from build123d import *

# Parameters (mm, degrees)
SKETCH4_W                         = 50
SKETCH4_H                         = 40
BOSS_EXTRUDE2_DEPTH               = 15
O_0_316_DIAMETER_HOLE1_AT_2_COUNT = 2
O_0_316_DIAMETER_HOLE1_AT_2_PITCH = 24
SKETCH10_W                        = 50
SKETCH10_H                        = 41.95
BOSS_EXTRUDE3_DEPTH               = 15
SKETCH12_W                        = 50
SKETCH12_H                        = 10
BOSS_EXTRUDE5_DEPTH               = 15
BOSS_EXTRUDE4_REACH               = 94.649
SKETCH11_W                        = 100
SKETCH11_H                        = 23.7
BOSS_EXTRUDE4_DIRECTION_2_DEPTH   = 25.4
O_0_316_DIAMETER_HOLE2_AT_2_COUNT = 2
O_0_316_DIAMETER_HOLE2_AT_2_PITCH = 25
O_0_316_DIAMETER_HOLE2_AT_3_COUNT = 2
O_0_316_DIAMETER_HOLE2_AT_3_PITCH = 50
O_0_316_DIAMETER_HOLE2_AT_4_COUNT = 2
O_0_316_DIAMETER_HOLE2_AT_4_PITCH = 75
CUT_EXTRUDE1_START                = -25.4
SKETCH13_R                        = 5.8
SKETCH13_R_2                      = 4.0132
CUT_EXTRUDE1_DEPTH                = 25.4
CHAMFER3_SIZE2                    = 25.4
CHAMFER3_SIZE                     = 14.664696837
FILLET1_R                         = 10


# Some blends are built 0.0001 mm under size
with BuildPart() as part:
    # Sketch4 → Boss-Extrude2 (new body)
    with BuildSketch(Plane(origin=(0, 0, 5), x_dir=(-1, 0, 0), z_dir=(0, 0, -1))):
        with Locations((6.635038983, -19.8)):
            Rectangle(SKETCH4_W, SKETCH4_H)
    extrude(amount=BOSS_EXTRUDE2_DEPTH)

    # Sketch9 → O (0.316) Diameter Hole1 (revolve, cut)
    with BuildSketch(Plane(origin=(-18.635038983, -19.8, 5), x_dir=(0, -1, 0), z_dir=(1, 0, 0))):
        Polygon((0, 0), (0, 15), (4.0132, 15), (4.0132, 6.350000732), (4.457235307, 0), align=None)
    o_0_316_diameter_hole1 = revolve(axis=Axis((-18.635038983, -19.8, 11.35), (0, 0, -1)), mode=Mode.SUBTRACT)

    # O (0.316) Diameter Hole1 at 2: O (0.316) Diameter Hole1 ×2
    with Locations(*[(i * O_0_316_DIAMETER_HOLE1_AT_2_PITCH, 0, 0) for i in range(1, O_0_316_DIAMETER_HOLE1_AT_2_COUNT)]):
        add(o_0_316_diameter_hole1, mode=Mode.SUBTRACT)

    # Sketch10 → Boss-Extrude3 (add)
    with BuildSketch(Plane(origin=(0, 0, -10), x_dir=(-1, 0, 0), z_dir=(0, 0, -1))):
        with Locations((6.635038983, -60.775)):
            Rectangle(SKETCH10_W, SKETCH10_H)
    extrude(amount=-BOSS_EXTRUDE3_DEPTH)

    # Sketch12 → Boss-Extrude5 (add)
    with BuildSketch(Plane.XY.offset(5)):
        with Locations((-6.635038983, -44.8)):
            Rectangle(SKETCH12_W, SKETCH12_H)
    extrude(amount=BOSS_EXTRUDE5_DEPTH)

    # Boss-Extrude4: up to this face of the body (flat: up to its plane)
    boss_extrude4_end = Plane(part.part.faces().sort_by_distance((-6.635038983, -19.8, 5))[0])
    # Sketch11 → Boss-Extrude4 (add, up to the picked face)
    with BuildSketch(Plane(origin=(0, 0, -10), x_dir=(-1, 0, 0), z_dir=(0, 0, -1)), mode=Mode.PRIVATE) as boss_extrude4_sk1:
        with Locations((-18.364961017, -69.9)):
            Rectangle(SKETCH11_W, SKETCH11_H)
    boss_extrude4_tool1 = split(extrude(boss_extrude4_sk1.sketch, amount=-BOSS_EXTRUDE4_REACH, mode=Mode.PRIVATE), bisect_by=boss_extrude4_end, keep=Keep.BOTH, mode=Mode.PRIVATE)
    add(boss_extrude4_tool1.solids().sort_by(Axis((18.364961, -69.9, -10), (0, 0, 1)))[0])

    # Sketch11 → Boss-Extrude4 direction 2 (add)
    with BuildSketch(Plane(origin=(0, 0, -10), x_dir=(-1, 0, 0), z_dir=(0, 0, -1))):
        with Locations((-18.364961017, -69.9)):
            Rectangle(SKETCH11_W, SKETCH11_H)
    extrude(amount=BOSS_EXTRUDE4_DIRECTION_2_DEPTH)

    # Sketch19 → O (0.316) Diameter Hole2 (revolve, cut)
    with BuildSketch(Plane(origin=(55.864961017, -69.9, -35.4), x_dir=(0, 1, 0), z_dir=(1, 0, 0))):
        Polygon((0, 0), (0, 55.4), (4.0132, 55.4), (4.0132, 6.349926268), (4.4572301, 0), align=None)
    o_0_316_diameter_hole2 = revolve(axis=Axis((55.864961017, -69.9, -41.75), (0, 0, 1)), mode=Mode.SUBTRACT)

    # O (0.316) Diameter Hole2 at 2: O (0.316) Diameter Hole2 ×2
    with Locations(*[(-i * O_0_316_DIAMETER_HOLE2_AT_2_PITCH, 0, 0) for i in range(1, O_0_316_DIAMETER_HOLE2_AT_2_COUNT)]):
        add(o_0_316_diameter_hole2, mode=Mode.SUBTRACT)

    # O (0.316) Diameter Hole2 at 3: O (0.316) Diameter Hole2 ×2
    with Locations(*[(-i * O_0_316_DIAMETER_HOLE2_AT_3_PITCH, 0, 0) for i in range(1, O_0_316_DIAMETER_HOLE2_AT_3_COUNT)]):
        add(o_0_316_diameter_hole2, mode=Mode.SUBTRACT)

    # O (0.316) Diameter Hole2 at 4: O (0.316) Diameter Hole2 ×2
    with Locations(*[(-i * O_0_316_DIAMETER_HOLE2_AT_4_PITCH, 0, 0) for i in range(1, O_0_316_DIAMETER_HOLE2_AT_4_COUNT)]):
        add(o_0_316_diameter_hole2, mode=Mode.SUBTRACT)

    # Sketch13 → Cut-Extrude1 (cut)
    # profile 1 of 4: a face of its own
    with BuildSketch(Plane.XY.offset(5).offset(CUT_EXTRUDE1_START)):
        with Locations((-19.135038983, -69.9)):
            Circle(SKETCH13_R)
        with Locations(Location((-19.135038983, -69.9, 0), (0, 0, 180))):
            Circle(SKETCH13_R_2, mode=Mode.SUBTRACT)
    # profile 2 of 4: a face of its own
    with BuildSketch(Plane.XY.offset(5).offset(CUT_EXTRUDE1_START)):
        with Locations((5.864961017, -69.9)):
            Circle(SKETCH13_R)
        with Locations(Location((5.864961017, -69.9, 0), (0, 0, 180))):
            Circle(SKETCH13_R_2, mode=Mode.SUBTRACT)
    # profile 3 of 4: a face of its own
    with BuildSketch(Plane.XY.offset(5).offset(CUT_EXTRUDE1_START)):
        with Locations((30.864961017, -69.9)):
            Circle(SKETCH13_R)
        with Locations(Location((30.864961017, -69.9, 0), (0, 0, 180))):
            Circle(SKETCH13_R_2, mode=Mode.SUBTRACT)
    # profile 4 of 4: a face of its own
    with BuildSketch(Plane.XY.offset(5).offset(CUT_EXTRUDE1_START)):
        with Locations((55.864961017, -69.9)):
            Circle(SKETCH13_R)
        with Locations(Location((55.864961017, -69.9, 0), (0, 0, 180))):
            Circle(SKETCH13_R_2, mode=Mode.SUBTRACT)
    extrude(amount=CUT_EXTRUDE1_DEPTH, mode=Mode.SUBTRACT)

    # Chamfer3
    chamfer3_edges = [part.edges().sort_by_distance(p)[0] for p in [
        (-6.635038983, -58.05, -10),
    ]]
    chamfer3_side = [part.faces().sort_by_distance(p)[0] for p in [
        (-6.635038983, -57.756706063, -10),
    ]]
    chamfer(chamfer3_edges, length=CHAMFER3_SIZE - 0.0001, length2=CHAMFER3_SIZE2 - 0.0001, reference=chamfer3_side[0])  # a hair under: the kernel refuses the full size

    # Fillet1
    fillet1_edges = [part.edges().sort_by_distance(p)[0] for p in [
        (-31.635038983, -81.75, -15.2),
        (68.364961017, -58.05, -15.2),
        (68.364961017, -81.75, -15.2),
        (18.364961017, 0.2, -2.5),
        (-31.635038983, 0.2, -2.5),
        (18.364961017, -58.05, -15.19995),
    ]]
    fillet(fillet1_edges, radius=FILLET1_R)

    # Chamfer2
    # the kernel refuses this chamfer: 2, 1.724779618 mm, written as the material it takes off along each edge
    with BuildSketch(Plane(origin=(18.519276683, -49.8, 5), x_dir=(-0.058004303634580846, 0.9983163330126716, 0), z_dir=(0, 0, 1))) as chamfer2_piece_1:
        with BuildLine():
            Line((1.793111056, 0), (0.030741404, 1.601811697))
            Line((0.030741404, 1.601811697), (-0.009191249, 1.60413187))
            ThreePointArc((-0.009191249, 1.60413187), (0.006496831, 0.80142144), (-0.039932653, 0.002320172))
            Line((-0.039932653, 0.002320172), (0.004703846, -0.03972246))
            ThreePointArc((0.004703846, -0.03972246), (0.895839611, 0.025445038), (1.790879262, -0.03993769))
            Line((1.790879262, -0.03993769), (1.793111056, 0))
        make_face()
    extrude(amount=19.48277764, mode=Mode.SUBTRACT)
    with BuildSketch(Plane(origin=(-31.635038983, -39.8, 5), x_dir=(0.9996219169112968, 0.0274958766105856, 0), z_dir=(0, 0, 1))) as chamfer2_piece_2:
        with BuildLine():
            Line((2.05734639, 0), (-0.11309431, -2.054235587))
            Line((-0.11309431, -2.054235587), (-0.153079186, -2.053135752))
            ThreePointArc((-0.153079186, -2.053135752), (-0.068258454, -1.026795659), (-0.039984877, 0.001099835))
            Line((-0.039984877, 0.001099835), (0.001099835, 0.039984877))
            ThreePointArc((0.001099835, 0.039984877), (1.028995329, 0.011711299), (2.058446225, 0.039984877))
            Line((2.058446225, 0.039984877), (2.05734639, 0))
        make_face()
    extrude(amount=20.143365976, mode=Mode.SUBTRACT)
    with BuildSketch(Plane(origin=(-31.635038983, -49.8, 5), x_dir=(0.9996219169112968, -0.027495876610585647, 0), z_dir=(0, 0, 1)), Plane(origin=(18.364961017, -39.8, 5), x_dir=(-0.9996219169112968, 0.027495876610585647, 0), z_dir=(0, 0, 1))) as chamfer2_piece_3:
        with BuildLine():
            Line((2.05734639, 0), (-0.11309431, 2.054235587))
            Line((-0.11309431, 2.054235587), (-0.153079186, 2.053135752))
            ThreePointArc((-0.153079186, 2.053135752), (-0.068258454, 1.026795659), (-0.039984877, -0.001099835))
            Line((-0.039984877, -0.001099835), (0.001099835, -0.039984877))
            ThreePointArc((0.001099835, -0.039984877), (1.028995329, -0.011711299), (2.058446225, -0.039984877))
            Line((2.058446225, -0.039984877), (2.05734639, 0))
        make_face()
    extrude(amount=20.143365976, mode=Mode.SUBTRACT)


solid = part.part
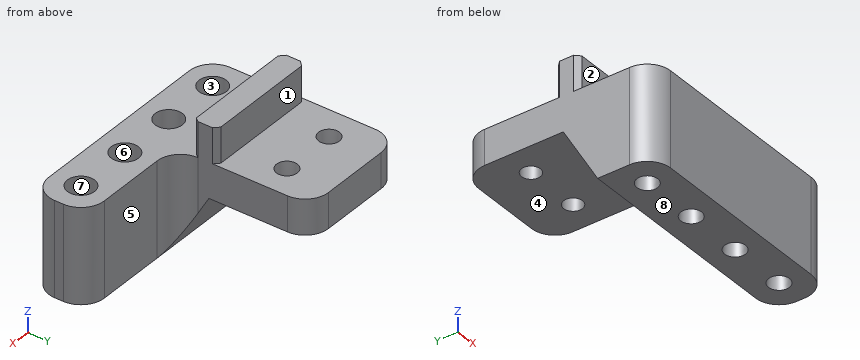
Source: CAD feature listing. Evaluate the final solid. Frame: model axes, mm. Face numbers are marked on the shaded views. A direction names the side the tool comes from. Give positions to 0.01 mm unless a question says otherwise; leave off trailing zeros. Write each loop counter-clockwise with the first axis right and the second up, starting at its lowest first coordinate (ties: lowest second). Pieces come first, ordered by that corner, then holes. Notation, with made-up numbers: (-19, 4) -> (1, 4) arc R29 cw to (1, 34) -> close; hole circle Ø1 at (69.25, 32). An arc over 180 degrees is marked (long way). Write item = value, one per line.
Q1. Mould query, pull axis Y, two halves, no side actions, for the marked faces 5, 6, 7 and 8. Classes: +Y half, -Y half, draft (parallel to the pull), parting line (faces both ways), or undercut.
Here are the results:
face_5 = +Y half
face_6 = undercut
face_7 = undercut
face_8 = draft
Q2. Cut plane D-D on z = -26.5. Return loops of the section in (x, y), then the cut area to 3 significant figures.
Here are the results:
outline = (-31.64, -71.75) arc R10 ccw to (-21.64, -81.75) -> (58.36, -81.75) arc R10 ccw to (68.36, -71.75) -> (68.36, -68.05) arc R10 ccw to (58.36, -58.05) -> (28.36, -58.05) arc R10 cw to (19.63, -52.91) -> (-31.64, -52.91) -> close; hole circle Ø8.03 at (-19.14, -69.9); hole circle Ø8.03 at (5.86, -69.9); hole circle Ø8.03 at (30.86, -69.9); hole circle Ø8.03 at (55.86, -69.9)
area = 2,380 mm²
Q3. Reachability of the marked faces 1, 2, 3 and 4 from +Z, -Z, +X, -X, +Y, -Y: full face, straight path, thin tool, end or side. Return the list, or none.
Here are the results:
face_1 = +Z, +X, -X, +Y
face_2 = +Z, +X, -X, -Y
face_3 = +Z
face_4 = -Z, +X, -X, +Y
Q4. First-contact query: pin 1 (8 mm diameter, centred on x = 20, z = 10.5, fed in from -Y); pin 2 (1 mm diameter, centred on y = -50, z = -17.5, fed in from +X); pin 3 (9.5 mm diameter, centred on x = -21, y = -68, fed in from +Z); pin 4 (6.5 mm diameter, centred on x = 55.86, y = -69.9, fed in from +Z). Flat tips, straight axial feed; report the tip coordinate or a pass-through.
Here are the results:
pin_1 = -49.8
pin_2 = 18.67
pin_3 = 5
pin_4 = through
Q5. Cut plane A-A on y = -19.8. Return loops of the section in (x, z), then the cut area to 3 significant figures.
Here are the results:
outline = (-31.64, -10) -> (-22.65, -10) -> (-22.65, -1.35) -> (-23.09, 5) -> (-31.64, 5) -> close; (-14.62, -10) -> (1.35, -10) -> (1.35, -1.35) -> (0.91, 5) -> (-14.18, 5) -> (-14.62, -1.35) -> close; (9.38, -10) -> (18.36, -10) -> (18.36, 5) -> (9.82, 5) -> (9.38, -1.35) -> close
area = 504 mm²
Q6. Line query: line 1 (X direction, y = -69.9, z = -24); line 2 (X direction, y = -73.5, z = -28.5); line 3 (X direction, y = -19, z = -6). Output: solid intervals per line, ascending. Write a range as from..to.
Here are the results:
line_1 = -31.64..-23.15, -15.12..1.85, 9.88..26.85, 34.88..51.85, 59.88..68.36
line_2 = -31.48..-20.91, -17.36..4.09, 7.64..29.09, 32.64..54.09, 57.64..68.21
line_3 = -31.64..-22.57, -14.7..1.43, 9.3..18.36
Q7. Cut plane C-C on z = -7. Return loops of the section in (x, y), then the cut area to 3 significant figures.
Here are the results:
outline = (-31.64, -71.75) arc R10 ccw to (-21.64, -81.75) -> (58.36, -81.75) arc R10 ccw to (68.36, -71.75) -> (68.36, -68.05) arc R10 ccw to (58.36, -58.05) -> (28.36, -58.05) arc R10 cw to (18.36, -48.05) -> (18.36, -9.8) arc R10 ccw to (8.36, 0.2) -> (-21.64, 0.2) arc R10 ccw to (-31.64, -9.8) -> close; hole circle Ø11.6 at (-19.14, -69.9); hole circle Ø8.03 at (-18.64, -19.8); hole circle Ø11.6 at (5.86, -69.9); hole circle Ø8.03 at (5.36, -19.8); hole circle Ø11.6 at (30.86, -69.9); hole circle Ø11.6 at (55.86, -69.9)
area = 4,670 mm²
